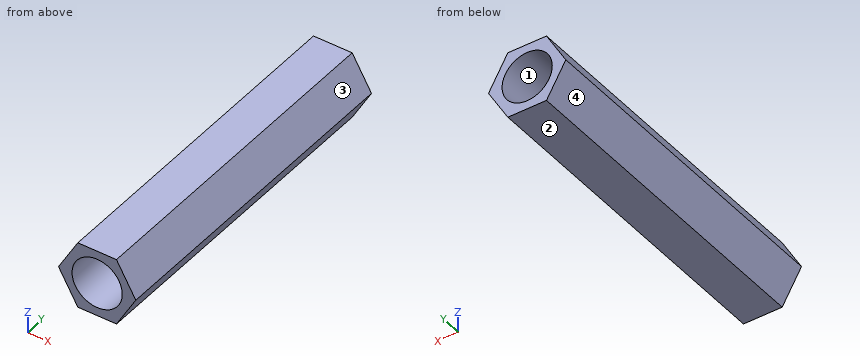
Autodesk Inventor part; units mm, degrees
ref_plane "YZ Plane" through (0, 0, 0) normal (1, 0, 0) x (0, 1, 0)
ref_plane "XZ Plane" through (0, 0, 0) normal (0, 1, 0) x (-1, 0, 0)
ref_plane "XY Plane" through (0, 0, 0) normal (0, 0, 1) x (1, 0, 0)
sketch "Эскиз1" plane through (0, 0, 0) normal (0, 1, 0) x (-1, 0, 0)
  line L0 (4.6188, 0) -> (2.3094, -4)
  line L1 (2.3094, -4) -> (-2.3094, -4)
  line L2 (-2.3094, -4) -> (-4.6188, 0)
  line L3 (-4.6188, 0) -> (-2.3094, 4)
  line L4 (-2.3094, 4) -> (2.3094, 4)
  line L5 (2.3094, 4) -> (4.6188, 0)
  circle A0 centre (0, 0) radius 3
  dimension "d0" = 8
  dimension "d1" = 8
  dimension "d2" = 6
extrude "Выдавливание1" add sketch "Эскиз1" along normal blind 40
thread "Резьба1"
properties part number "stoyka_M6_40mm" material "Сталь нержавеющая, 440C"
Geometry check sheet. Reference: the model listing, model coordinates, mm. Face numbers are marked on the shaded views. Coordinates: 2 decimals unless noted, no trailing zeros. Write each loop counter-clockwise with the first axis right and the second up, starting at its lowest first coordinate (ties: lowest second). Pieces come first, ordered by that corner, then holes. Notation, with made-up numbers: (-25.5, 44.25) -> (11.5, 44.25) arc R9 cw to (11.5, 60.25) -> close; hole circle Ø6 at (75, 8). An arc over 180 degrees is marked (long way). Use CSV: the item, a comma, the result in double quotes. Start each with the question number.
Item 1: Cross-section at D-D, the plane z = 3.5. Record the cut outline in (x, y).
Item 2: Depth check by flat-ended pin: pin 1 Ø2 at (y, z) = (32, -3) entering from -X; pin 2 Ø1.5 at (y, z) = (32, 2.5) entering from +X; pin 3 Ø5 at (x, y) = (-3, 13.5) entering from +Z. Enter the tip coordinate at first touch or a pass-through.
Item 3: Mould release check, pull along X, two halves, no side actions. Record for the marked faces 1, 2, 3 and 4: released by +X, released by -X, zero draft, split by the parting line, or undercut.
Item 4: Cross-section at A-A, the plane x = 0. Record the cut outline in (y, z), plus the area to 3 significant figures.
Item 5: Cross-section at B-B, the plane y = 28. Record the cut outline in (x, z), plus the area to 3 significant figures.
Item 6: Cross-section at C-C, the plane z = 1.5. Record the cut outline in (x, y).
Item 7: Thickness scan on line 1 (Z direction, x = 0, y = 26); line 2 (Z direction, x = -2.5, y = 31); line 3 (X direction, y = 14, z = -1). Record the ranges inside material, lowest first.
Answers:
1,outline,"(-2.6, 0) -> (2.6, 0) -> (2.6, 40) -> (-2.6, 40) -> close"
2,pin 1,"x = -3.46"
2,pin 2,"x = 3.61"
2,pin 3,"z = 4"
3,face 1,"undercut"
3,face 2,"zero draft"
3,face 3,"released by +X"
3,face 4,"released by -X"
4,outline,"(0, -4) -> (40, -4) -> (40, -3) -> (0, -3) -> close; (0, 3) -> (40, 3) -> (40, 4) -> (0, 4) -> close"
4,area,"80.0 mm^2"
5,outline,"(-4.62, 0) -> (-2.31, -4) -> (2.31, -4) -> (4.62, 0) -> (2.31, 4) -> (-2.31, 4) -> close; hole circle Ø6 at (0, 0)"
5,area,"27.2 mm^2"
6,outline,"(-3.75, 0) -> (-2.6, 0) -> (-2.6, 40) -> (-3.75, 40) -> close; (2.6, 0) -> (3.75, 0) -> (3.75, 40) -> (2.6, 40) -> close"
7,line 1,"-4 to -3, 3 to 4"
7,line 2,"-3.67 to -1.66, 1.66 to 3.67"
7,line 3,"-4.04 to -2.83, 2.83 to 4.04"
